Could you check a few things on this model? Use its own coordinates, in mm. Face numbers are marked on the shaded views. Coordinates: 2 decimals unless noted, no trailing zeros. Write each loop counter-clockwise with the first axis right and the second up, starting at its lowest first coordinate (ties: lowest second). Pieces come first, ordered by that corner, then holes. Notation, with made-up numbers: (68.25, 85.5) - (88.25, 85.5) arc R19 cw to (88.25, 114.5) - close; hole circle Ø7 at (51.5, 52). An arc over 180 degrees is marked (long way). Answer as a JSON object with one key per item and string values. Group by question number.
1) If we section it at C-C (z = -12): Write out the boundary of the cut face in (x, y), plus the area to 3 significant figures.
2) Will these pins go through, and if not, where does the flat tip stop? pin 1 Ø4 at (x, z) = (0, 0) entering from -Y; pin 2 Ø2 at (x, y) = (4.5, 3) entering from +Z; pin 3 Ø3 at (x, z) = (-8.49, -8.49) entering from -Y.
3) If we section it at A-A (x = 0): Write out the boundary of the cut face in (y, z), plus the area to 3 significant figures.
4) If we section it at B-B (x = -7.5): Write out the boundary of the cut face in (y, z).
5) Please list where these lines run through material, in increasing order: line 1 along X through (y, z) = (1.3, -8); line 2 along X through (y, z) = (1.65, 1); line 3 along Z through (x, y) = (-6.75, 2.85).
6) If we section it at D-D (x = 8.25): Write out the boundary of the cut face in (y, z), plus the area to 3 significant figures.
7) We'd pull the mould along X, two halves only. Please class the marked faces 1, 2 and 3: released by +X, released by -X, zero draft, split by the parting line, or undercut.
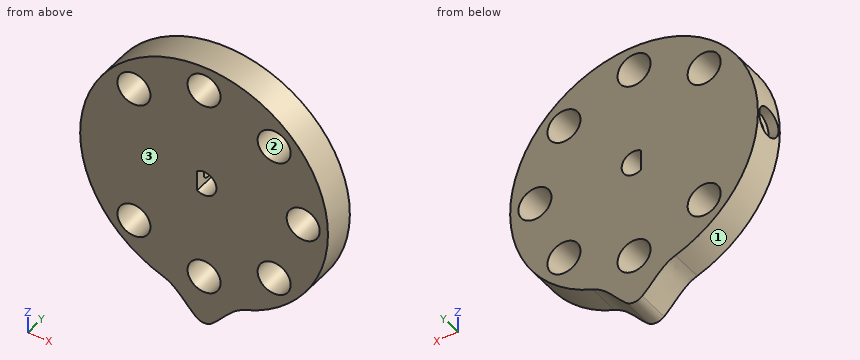
Autodesk Inventor part; units mm, degrees
ref_plane "Work Plane1" through (-15, 0, 0) normal (1, 0, 0) x (0, 1, 0)
ref_plane "XZ Plane" through (0, 0, 0) normal (0, 1, 0) x (-1, 0, 0)
ref_plane "XY Plane" through (0, 0, 0) normal (0, 0, 1) x (1, 0, 0)
sketch "Sketch1" plane through (0, 0, 0) normal (0, 1, 0) x (-1, 0, 0)
  arc A0 (0.8292, 1.25) -> (0.8292, -1.25) centre (0, 0) ccw
  line L0 (0.8292, 1.25) -> (0.8292, -1.25)
  circle A1 centre (0, 0) radius 15 construction
  circle A2 centre (0, 0) radius 18 construction
  line L1 (0, -15) -> (0, -18) construction
  arc A3 (-1, -17.618) -> (1, -17.618) centre (0, -16.5) ccw
  spline S0 degree 3 poles (1, -17.618) (2.3167, -16.4404) (3.2766, -14.7515) (5, -14.1421) knots 0 0 0 0 1 1 1 1
  spline S1 degree 3 poles (-1, -17.618) (-2.3167, -16.4404) (-3.2766, -14.7515) (-5, -14.1421) knots 0 0 0 0 1 1 1 1
  arc A4 (5, -14.1421) -> (-5, -14.1421) centre (0, 0) ccw
  line L2 (0, 0) -> (13.7006, 0) construction
  line L3 (0, 0) -> (0, -3.6917) construction
  circle A5 centre (-12, 0) radius 2
  circle A6 centre (-8.4853, -8.4853) radius 2
  circle A7 centre (0, -12) radius 2
  circle A8 centre (8.4853, -8.4853) radius 2
  circle A9 centre (12, 0) radius 2 construction
  circle A10 centre (8.4853, 8.4853) radius 2
  circle A11 centre (0, 12) radius 2
  circle A12 centre (-8.4853, 8.4853) radius 2
  dimension "d50" = 36
  dimension "d0" = 3
  dimension "d1" = 2.5
  dimension "d2" = 30
  dimension "d7" = 5
  dimension "d8" = 1
  dimension "d9" = 5
  dimension "d29" = 12
  dimension "d30" = 4
  dimension "d33" = 360
extrude "Extrusion1" add sketch "Sketch1" along normal blind 4
ref_plane "Work Plane1" through (-15, 0, 0) normal (1, 0, 0) x (0, 1, 0)
ref_plane "Work Plane2" through (-15, 0, 0) normal (1, 0, 0) x (0, 1, 0)
sketch "Sketch6" plane through (-15, 0, 0) normal (1, 0, 0) x (0, 1, 0)
  line L0 (4, -14.1421) -> (4, 15) construction
  line L1 (0, 15) -> (0, -14.1421) construction
  line L2 (0, 0) -> (4, 0) construction
  circle A0 centre (2, 0) radius 1.75
  dimension "d41" = 3.5
extrude "Extrusion6" cut sketch "Sketch6" along normal blind 1.2
sketch "Sketch8" plane through (-15, 0, 0) normal (1, 0, 0) x (0, 1, 0)
  circle A0 centre (2, 0) radius 0.8
  point P0 (0, 0)
  dimension "d47" = 1.6
extrude "Extrusion8" cut sketch "Sketch8" along normal up to surface (14.1708 mm away)
properties part number "servo horn"
Here are the results:
{
 "1": {"outline": "(-9, 0) - (-2, 0) - (-2, 4) - (-9, 4) - close; (2, 0) - (9, 0) - (9, 4) - (2, 4) - close", "area": "56.0 mm²"},
 "2": {"pin 1": "stops at y = 0", "pin 2": "stops at z = 14.59", "pin 3": "passes through"},
 "3": {"outline": "(0, -18) - (4, -18) - (4, -14) - (0, -14) - close; (0, -10) - (4, -10) - (4, -1.5) - (0, -1.5) - close; (0, 1.5) - (4, 1.5) - (4, 10) - (0, 10) - close; (0, 14) - (4, 14) - (4, 15) - (0, 15) - close", "area": "88.0 mm²"},
 "4": {"outline": "(0, -12.99) - (4, -12.99) - (4, -10.23) - (0, -10.23) - close; (0, -6.74) - (4, -6.74) - (4, 6.74) - (0, 6.74) - close; (0, 10.23) - (4, 10.23) - (4, 12.99) - (0, 12.99) - close; hole circle Ø1.6 at (2, 0)"},
 "5": {"line 1": "x = -12.69 to -10.43, -6.55 to 6.55, 10.43 to 12.69", "line 2": "x = -13.8 to -0.83, 1.12 to 10.27, 13.73 to 14.97", "line 3": "z = -13.4 to -9.48, -7.49 to 7.49, 9.48 to 13.4"},
 "6": {"outline": "(0, -12.53) - (4, -12.53) - (4, -10.47) - (0, -10.47) - close; (0, -6.5) - (4, -6.5) - (4, 6.5) - (0, 6.5) - close; (0, 10.47) - (4, 10.47) - (4, 12.53) - (0, 12.53) - close", "area": "68.4 mm²"},
 "7": {"face 1": "split by the parting line", "face 2": "undercut", "face 3": "zero draft"}
}
